For this review, take the finished solid that the model builds, in its own axes (mm). A direction names the side the tool comes from. Round coordinates to 2 decimals unless told otherwise and drop trailing zeros. Loops run counter-clockwise (first coordinate to the right, second up) from the corner with the lowest first, then second, coordinate; pieces in that order, holes last.
1) Take a section at A-A (x = 0). State the section outline as (y, z) points.
2) Take a section at C-C (z = -117.5). State the section outline as (x, y) points, then the cut area to 3 significant figures.
3) Take a section at B-B (z = -76.5). State the section outline as (x, y) points, then the cut area to 3 significant figures.
4) Wall thickness on L1, parallel to Z at x = -21, y = 6; L2, parallel to X at y = 5, z = -99; L3, parallel to X at y = 5.25, z = -138: over which ranges is each line inside the solid? List them lowest first.
5) Tool access review of faces 4 (the cylindrical face through (43.482, 4.93, -152.242)), 5 (the flat face through (0, 10, 2)), 6 (the cylindrical face through (-48.549, 5.07, -115.954)): name each direction out of +Z, -Z, +X, -X, +Y, -Y from which nothing blocks a thin tool from reaching the whole face with its end or side.
6) Insertion check: pin 1 (6 mm diameter, centred on y = 7.5, z = -94.5, fed in from -X); pin 2 (2 mm diameter, centred on x = 61.5, z = -68, fed in from -Y); pin 3 (3 mm diameter, centred on x = -4.5, y = 3.5, fed in from +Z); pin 4 (4 mm diameter, centred on x = 42.5, y = 1, fed in from -Z). Each pin has a flat end and moves straight along its axis. Give the tip position at first contact, or say it passes through.
7) Mouldability with a two-part tool opening along Z and no side actions: class faces 1 (the cylindrical face through (-55.5, 4.93, -161.08)), 2 (the flat face through (0, 5, 27.5)), 3 (the cylindrical face through (49.324, 4.93, -136.395)) as pulls with the +Z half, pulls with the -Z half, needs draft (parallel to the pull), parting line crosses it, or undercut.
8) Take a section at D-D (x = 20.5). State the section outline as (y, z) points.
```python
from build123d import *

# Parameters (mm, degrees)
EXTRUDE_1_DEPTH     = 10
CUT_EXTRUDE_1_REACH = 193.075
SKETCH_2_R          = 2.15
FILLET_1_R          = 1


with BuildPart() as part:
    # 草图1 → 凸台-拉伸1 (new body)
    with BuildSketch(Plane(origin=(0, 0, 0), x_dir=(1, 0, 0), z_dir=(0, 1, 0))):
        with BuildLine():
            Line((-23, 0), (23, 0))
            Line((23, 0), (50.280437597, 32.511559514))
            ThreePointArc((50.280437597, 32.511559514), (50.971701439, 33.798064087), (51.092639409, 35.25350688))
            Line((51.092639409, 35.25350688), (36.048986901, 157.774224452))
            ThreePointArc((36.048986901, 157.774224452), (37.845160212, 160.483167311), (40.799539436, 159.128083042))
            ThreePointArc((40.799539436, 159.128083042), (43.514050375, 152.141566893), (45.33631399, 144.871124481))
            Line((45.33631399, 144.871124481), (46.228669547, 142.01495601))
            ThreePointArc((46.228669547, 142.01495601), (46.250999528, 141.886354071), (46.239284003, 141.756354712))
            Line((46.239284003, 141.756354712), (45.962164319, 140.52161209))
            Line((45.962164319, 140.52161209), (46.010409332, 140.218889241))
            ThreePointArc((46.010409332, 140.218889241), (46.065188715, 139.673724891), (46.11498752, 139.128083042))
            ThreePointArc((46.11498752, 139.128083042), (49.390100294, 136.400799361), (52.087350199, 139.700690708))
            Line((52.087350199, 139.700690708), (51.968804209, 140.828580455))
            Line((51.968804209, 140.828580455), (51.095150293, 141.978953599))
            ThreePointArc((51.095150293, 141.978953599), (51.00671283, 142.166476528), (51.001947429, 142.37375249))
            Line((51.001947429, 142.37375249), (51.517960099, 145.118075635))
            Line((51.517960099, 145.118075635), (50.997668008, 150.068324212))
            ThreePointArc((50.997668008, 150.068324212), (51.882837828, 151.945152782), (53.956331039, 152.026620552))
            Line((53.956331039, 152.026620552), (59.401206432, 149.008476838))
            ThreePointArc((59.401206432, 149.008476838), (60.04962118, 148.434807928), (60.394841558, 147.640855414))
            Line((60.394841558, 147.640855414), (81.828137025, 37.376109146))
            ThreePointArc((81.828137025, 37.376109146), (81.874721206, 33.817543133), (80.672119228, 30.468019192))
            Line((80.672119228, 30.468019192), (47.950739183, -26.207073541))
            ThreePointArc((47.950739183, -26.207073541), (46.63822592, -27.519586803), (44.845299462, -28))
            Line((44.845299462, -28), (10.707106781, -28))
            ThreePointArc((10.707106781, -28), (10.515765065, -27.961939766), (10.353553391, -27.853553391))
            Line((10.353553391, -27.853553391), (10, -27.5))
            Line((10, -27.5), (-10, -27.5))
            Line((-10, -27.5), (-10.353553391, -27.853553391))
            ThreePointArc((-10.353553391, -27.853553391), (-10.515765065, -27.961939766), (-10.707106781, -28))
            Line((-10.707106781, -28), (-44.845299462, -28))
            ThreePointArc((-44.845299462, -28), (-45.845299462, -27.732050808), (-46.577350269, -27))
            Line((-46.577350269, -27), (-54.72793721, -12.882769307))
            Line((-54.72793721, -12.882769307), (-80.672119228, 30.468019192))
            ThreePointArc((-80.672119228, 30.468019192), (-81.874721206, 33.817543133), (-81.828137025, 37.376109146))
            Line((-81.828137025, 37.376109146), (-60.216890167, 148.556335961))
            ThreePointArc((-60.216890167, 148.556335961), (-55.407693084, 161.241250242), (-46.635305706, 171.589228142))
            ThreePointArc((-46.635305706, 171.589228142), (-43.253111024, 171.912359616), (-41.738335903, 168.871124481))
            ThreePointArc((-41.738335903, 168.871124481), (-41.556322934, 156.551185491), (-37.633288365, 144.871124481))
            Line((-37.633288365, 144.871124481), (-51.176674229, 34.569098196))
            ThreePointArc((-51.176674229, 34.569098196), (-51.109221395, 33.75732882), (-50.723670812, 33.03978429))
            Line((-50.723670812, 33.03978429), (-23, 0))
        make_face()
    extrude(amount=EXTRUDE_1_DEPTH)

    # 草图2 → 切除-拉伸1 (cut, up to next)
    with BuildSketch(Plane(origin=(0, 10, 0), x_dir=(1, 0, 0), z_dir=(0, 1, 0)), mode=Mode.PRIVATE) as cut_extrude_1_sk1:
        with Locations(Location((0, -23.5, 0), (0, 0, 270))):
            Circle(SKETCH_2_R)
    cut_extrude_1_tool1 = extrude(cut_extrude_1_sk1.sketch, amount=-CUT_EXTRUDE_1_REACH, mode=Mode.PRIVATE) & part.part
    # 草图2 → 切除-拉伸1 (cut, up to next)
    with BuildSketch(Plane(origin=(0, 10, 0), x_dir=(1, 0, 0), z_dir=(0, 1, 0)), mode=Mode.PRIVATE) as cut_extrude_1_sk2:
        with Locations(Location((0, -15.5, 0), (0, 0, 270))):
            Circle(SKETCH_2_R)
    cut_extrude_1_tool2 = extrude(cut_extrude_1_sk2.sketch, amount=-CUT_EXTRUDE_1_REACH, mode=Mode.PRIVATE) & part.part
    # 草图2 → 切除-拉伸1 (cut, up to next)
    with BuildSketch(Plane(origin=(0, 10, 0), x_dir=(1, 0, 0), z_dir=(0, 1, 0)), mode=Mode.PRIVATE) as cut_extrude_1_sk3:
        with BuildLine():
            Line((-44.965311668, 137.162976975), (-44.804514377, 135.345756555))
            Line((-44.804514377, 135.345756555), (-45.277917872, 134.596824083))
            ThreePointArc((-45.277917872, 134.596824083), (-45.354871903, 134.349709989), (-45.297959002, 134.097225891))
            Line((-45.297959002, 134.097225891), (-44.452214101, 132.486513242))
            ThreePointArc((-44.452214101, 132.486513242), (-42.963225579, 126.529787442), (-40.580117827, 120.871124481))
            Line((-40.580117827, 120.871124481), (-43.035809045, 100.871124481))
            ThreePointArc((-43.035809045, 100.871124481), (-48.604809202, 116.175489254), (-50.95898566, 132.29055044))
            Line((-50.95898566, 132.29055044), (-50.219666113, 133.859541555))
            ThreePointArc((-50.219666113, 133.859541555), (-50.172028753, 134.06484851), (-50.213221053, 134.271545048))
            Line((-50.213221053, 134.271545048), (-51.032139087, 136.160541322))
            ThreePointArc((-51.032139087, 136.160541322), (-51.021228549, 137.124454778), (-50.998704156, 138.08816679))
            ThreePointArc((-50.998704156, 138.08816679), (-47.997070546, 140.99999857), (-45.001129375, 138.082310248))
            ThreePointArc((-45.001129375, 138.082310248), (-44.985863781, 137.622540629), (-44.965311668, 137.162976975))
        make_face()
    cut_extrude_1_tool3 = extrude(cut_extrude_1_sk3.sketch, amount=-CUT_EXTRUDE_1_REACH, mode=Mode.PRIVATE) & part.part
    add(cut_extrude_1_tool1.solids().sort_by_distance((0, 10, 23.5))[0], mode=Mode.SUBTRACT)
    add(cut_extrude_1_tool2.solids().sort_by_distance((0, 10, 15.5))[0], mode=Mode.SUBTRACT)
    add(cut_extrude_1_tool3.solids().sort_by_distance((-45.998672, 10, -122.997327))[0], mode=Mode.SUBTRACT)

    # 圆角1
    fillet_1_edges = [part.edges().sort_by_distance(p)[0] for p in [
        (-40.580117827, 5, -120.871124481),
        (-37.633288365, 5, -144.871124481),
    ]]
    fillet(fillet_1_edges, radius=FILLET_1_R)


solid = part.part
```
Response:
1. outline: (0, 0) - (10, 0) - (10, 13.35) - (0, 13.35) - close; (0, 17.65) - (10, 17.65) - (10, 21.35) - (0, 21.35) - close; (0, 25.65) - (10, 25.65) - (10, 27.5) - (0, 27.5) - close
2. outline: (-66.25, 0) - (-48.93, 0) - (-48.93, 10) - (-66.25, 10) - close; (40.99, 0) - (66.25, 0) - (66.25, 10) - (40.99, 10) - close
2. area: 426 mm2
3. outline: (-74.22, 0) - (-46.03, 0) - (-46.03, 10) - (-74.22, 10) - close; (46.03, 0) - (74.22, 0) - (74.22, 10) - (46.03, 10) - close
3. area: 564 mm2
4. L1: z = 0 to 28
4. L2: x = -69.85 to -43.27, 43.27 to 69.85
4. L3: x = -62.27 to -51, -45 to -38.48, 38.48 to 46.44, 51.76 to 62.27
5. face 4: -Z, +Y, -Y
5. face 5: +Z, -Z, +X, -X, +Y
5. face 6: +Y, -Y
6. pin 1: stops at x = -71.31
6. pin 2: stops at y = 0
6. pin 3: stops at z = 27.5
6. pin 4: stops at z = -159.62
7. face 1: pulls with the -Z half
7. face 2: pulls with the +Z half
7. face 3: undercut
8. outline: (0, 0) - (10, 0) - (10, 28) - (0, 28) - close
